CAD build for the part. Positions are in the model's coordinates, mm. Face numbers are marked on the shaded views. A direction names the side the tool comes from. Round coordinates to 2 decimals unless told otherwise and drop trailing zeros. Order: outer loops, then holes, each group sorted by start corner. A loop starts at its lowest first (then second) coordinate and runs counter-clockwise, first axis right, second up. Notation, with made-up numbers: (1, 60.5) -> (29, 60.5) arc R17 ccw to (29, 70.5) -> close; hole circle Ø2 at (30, 45). An arc over 180 degrees is marked (long way). Return JSON: item names as keys, results as strings. Group by question number.
Q1. Cut at A-A (y = 8). Write the cut outline in (x, z), then the cut area to 3 significant figures.
Q2. Flat gauge pins, fed straight in: pin 1 (2.5 mm diameter, centred on x = 43, z = -48, fed in from +Y); pin 2 (4.5 mm diameter, centred on y = 27.5, z = 47.5, fed in from +X); pin 3 (6 mm diameter, centred on x = -21, z = 33, fed in from +Y). Where does each tip first touch, or does it go through?
Q3. Cut at C-C (z = 13). Write the cut outline in (x, y), then the cut area to 3 significant figures.
Q4. Probe line 1 along X through (y, z) = (-13, -21); line 2 along Y through (x, z) = (16.5, 22). List the from-to ranges inside material, lowest first.
Q5. Cut at B-B (x = 35.5). Write the cut outline in (y, z).
Q6. Which spindle directions (+Z, -Z, +X, -X, +Y, -Y) get a long thin tool onto all of the face, cutting with end or side? Do the marked faces 4, 5 and 6. Say none if no direction does.
Q7. Mould opens along Z. For the marked faces 1, 2 and 3 say: +Z half, -Z half, draft (parallel to the pull), parting line (faces both ways), or undercut.
Q8. Cut at D-D (y = 29). Count the separate pieces of the cut face and the enclosed holes in it, then the cut area to 3 significant figures.
from build123d import *

# Parameters (mm, degrees)
SKETCH1_W           = 100
SKETCH1_H           = 100
BOSS_EXTRUDE1_DEPTH = 25
SKETCH4_W           = 80
SKETCH4_H           = 80
CUT_EXTRUDE2_DEPTH  = 40
SKETCH5_R           = 7.5
CUT_EXTRUDE3_DEPTH  = 100
BOSS_EXTRUDE4_DEPTH = 10
BOSS_EXTRUDE5_DEPTH = 10
BOSS_EXTRUDE6_START = -90
SKETCH9_W           = 32.5
SKETCH9_H           = 8.660254038
BOSS_EXTRUDE6_DEPTH = 10
SKETCH11_W          = 32.5
SKETCH11_H          = 8.660254038
BOSS_EXTRUDE8_DEPTH = 10


with BuildPart() as part:
    # Sketch1 → Boss-Extrude1 (new body, symmetric)
    with BuildSketch(Plane(origin=(0, 0, 0), x_dir=(1, 0, 0), z_dir=(0, 1, 0))):
        Rectangle(SKETCH1_W, SKETCH1_H)
    extrude(amount=BOSS_EXTRUDE1_DEPTH, both=True)

    # Sketch4 → Cut-Extrude2 (cut)
    with BuildSketch(Plane(origin=(0, 25, 0), x_dir=(1, 0, 0), z_dir=(0, 1, 0))):
        Rectangle(SKETCH4_W, SKETCH4_H)
    extrude(amount=-CUT_EXTRUDE2_DEPTH, mode=Mode.SUBTRACT)

    # Sketch5 → Cut-Extrude3 (cut)
    with BuildSketch(Plane.XY.offset(50)):
        with Locations((0, 25)):
            Circle(SKETCH5_R)
    extrude(amount=-CUT_EXTRUDE3_DEPTH, mode=Mode.SUBTRACT)

    # Sketch7 → Boss-Extrude4 (add)
    with BuildSketch(Plane.ZY.offset(50)):
        Polygon((40, 33.660254038), (35, 25), (45, 25), align=None)
        Polygon((30, 33.660254038), (25, 25), (35, 25), align=None)
        Polygon((20, 33.660254038), (15, 25), (25, 25), align=None)
        Polygon((10, 33.660254038), (5, 25), (15, 25), align=None)
        Polygon((0, 33.660254038), (-5, 25), (5, 25), align=None)
        Polygon((-10, 33.660254038), (-15, 25), (-5, 25), align=None)
        Polygon((-20, 33.660254038), (-25, 25), (-15, 25), align=None)
        Polygon((-30, 33.660254038), (-35, 25), (-25, 25), align=None)
        Polygon((-40, 33.660254038), (-45, 25), (-35, 25), align=None)
    extrude(amount=-BOSS_EXTRUDE4_DEPTH)

    # Sketch8 → Boss-Extrude5 (add)
    with BuildSketch(Plane(origin=(50, 0, 0), x_dir=(0, 0, -1), z_dir=(1, 0, 0))):
        Polygon((40, 33.660254038), (35, 25), (45, 25), align=None)
        Polygon((30, 33.660254038), (25, 25), (35, 25), align=None)
        Polygon((20, 33.660254038), (15, 25), (25, 25), align=None)
        Polygon((10, 33.660254038), (5, 25), (15, 25), align=None)
        Polygon((0, 33.660254038), (-5, 25), (5, 25), align=None)
        Polygon((-10, 33.660254038), (-15, 25), (-5, 25), align=None)
        Polygon((-20, 33.660254038), (-25, 25), (-15, 25), align=None)
        Polygon((-30, 33.660254038), (-35, 25), (-25, 25), align=None)
        Polygon((-40, 33.660254038), (-45, 25), (-35, 25), align=None)
    extrude(amount=-BOSS_EXTRUDE5_DEPTH)

    # Sketch9 → Boss-Extrude6 (add)
    with BuildSketch(Plane.XY.offset(50).offset(BOSS_EXTRUDE6_START)):
        with Locations((-23.75, 29.330127019)):
            Rectangle(SKETCH9_W, SKETCH9_H)
        with Locations((23.75, 29.330127019)):
            Rectangle(SKETCH9_W, SKETCH9_H)
    extrude(amount=-BOSS_EXTRUDE6_DEPTH)

    # Sketch11 → Boss-Extrude8 (add)
    with BuildSketch(Plane.XY.offset(50)):
        with Locations((-23.75, 29.330127019)):
            Rectangle(SKETCH11_W, SKETCH11_H)
        with Locations((23.75, 29.330127019)):
            Rectangle(SKETCH11_W, SKETCH11_H)
    extrude(amount=-BOSS_EXTRUDE8_DEPTH)


solid = part.part
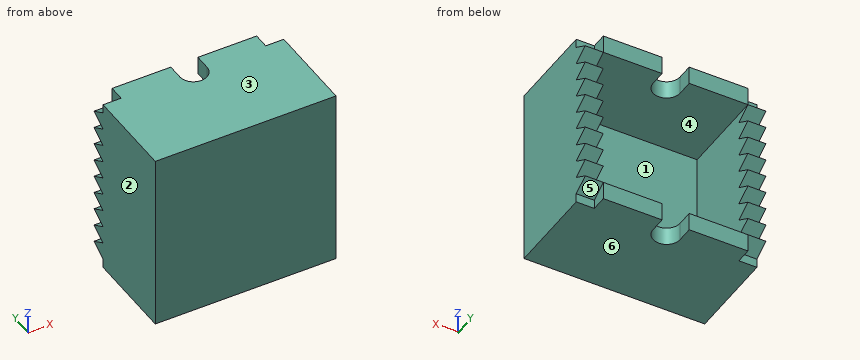
Solution:
{
 "1": {"outline": "(-50, -50) -> (50, -50) -> (50, 50) -> (-50, 50) -> close; hole (-40, -40) -> (40, -40) -> (40, 40) -> (-40, 40) -> close", "area": "3,600 mm²"},
 "2": {"pin 1": "stops at y = 25", "pin 2": "stops at x = 40", "pin 3": "stops at y = -15"},
 "3": {"outline": "(-50, -25) -> (50, -25) -> (50, 28.46) -> (40, 28.46) -> (40, -15) -> (-40, -15) -> (-40, 28.46) -> (-50, 28.46) -> close", "area": "1,870 mm²"},
 "4": {"line 1": "x = -50 to -40, 40 to 50", "line 2": "y = -25 to -15"},
 "5": {"outline": "(-25, -50) -> (33.66, -50) -> (33.66, -40) -> (-15, -40) -> (-15, 40) -> (33.66, 40) -> (33.66, 50) -> (-25, 50) -> close"},
 "6": {"face 4": "+Y", "face 5": "-Z, +X, +Y", "face 6": "-Z, +X, -X, +Y, -Y"},
 "7": {"face 1": "undercut", "face 2": "draft", "face 3": "+Z half"},
 "8": {"separate pieces": "18", "enclosed holes": "0", "area": "2,270 mm²"}
}
